Can you work these out from the model? Positions are in its coordinate system, mm. Coordinates: 2 decimals unless noted, no trailing zeros. Write each loop counter-clockwise with the first axis right and the second up, starting at its lowest first coordinate (ties: lowest second). Pieces come first, ordered by that corner, then holes. Notation, with made-up numbers: (51.25, -1) - (75.25, -1) arc R6 ccw to (75.25, 3) - close; hole circle Ø2 at (61, 72.5). An arc over 180 degrees is marked (long way). Use one line per item in the form item = value. Start each with the question number.
(1) If we section it at C-C on z = -33.5: Please give me the cut outline in (x, y).
(2) If I drill on probe 1 along X at (y, z) = (1.05, -12.5); probe 2 along X at (y, z) = (0.9, -21); probe 3 along X at (y, z) = (2.1, -23.35), over which ranges is the centre line in solid material (lowest first)? Write a range as from..to.
(3) For pin 1 Ø0.9 at (x, y) = (55, 2) entering from -Z, with a flat end and sliding along its axis, tell me the tip position at first contact or that it passes through.
(4) If we section it at B-B on z = -12.5: Please give me the cut outline in (x, y).
(5) If we section it at A-A on x = 47: Please give me the cut outline in (y, z), then the cut area to 4 significant figures.
(6) If we section it at D-D on x = 32: Please give me the cut outline in (y, z).
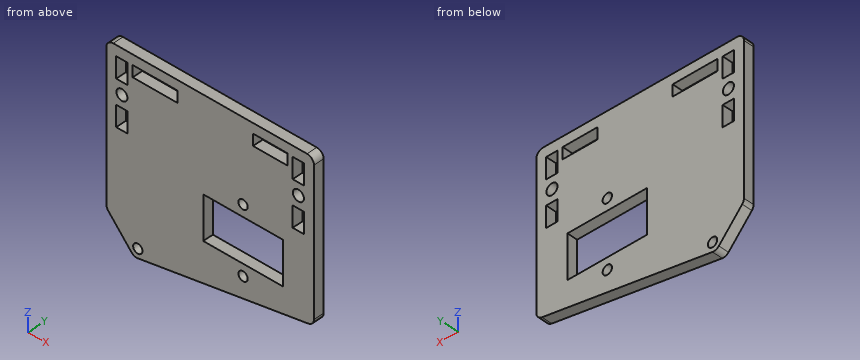
```python
from build123d import *

# Parameters (mm, degrees)
BOSS_EXTRUDE1_DEPTH = 3
SKETCH2_R           = 1.35
SKETCH2_R_2         = 1.6
SKETCH2_W           = 3
SKETCH2_H           = 6
SKETCH2_W_2         = 13
SKETCH2_H_2         = 3
SKETCH2_W_3         = 10
SKETCH2_W_4         = 23
SKETCH2_H_3         = 12.5
MAIN_HOLES_DEPTH    = 4
SKETCH3_W           = 0.15
SKETCH3_H           = 6
SKETCH3_W_2         = 10
SKETCH3_H_2         = 0.15
SKETCH3_W_3         = 13
TOLERANCE_DEPTH     = 4


with BuildPart() as part:
    # Sketch1 → Boss-Extrude1 (new body)
    with BuildSketch(Plane(origin=(0, 0, 0), x_dir=(1, 0, 0), z_dir=(0, 1, 0))):
        with BuildLine():
            Line((58.341082867, 45.287120273), (9.096557402, 53.810211219))
            ThreePointArc((9.096557402, 53.810211219), (8.095316223, 53.72741672), (7.260655898, 53.168237885))
            Line((7.260655898, 53.168237885), (0.505181363, 45.568329033))
            ThreePointArc((0.505181363, 45.568329033), (0.130556597, 44.95036247), (0, 44.239601355))
            Line((0, 44.239601355), (0, 2))
            ThreePointArc((0, 2), (0.585786438, 0.585786438), (2, 0))
            Line((2, 0), (58, 0))
            ThreePointArc((58, 0), (59.414213562, 0.585786438), (60, 2))
            Line((60, 2), (60, 43.316419261))
            ThreePointArc((60, 43.316419261), (59.530059759, 44.604408831), (58.341082867, 45.287120273))
        make_face()
    extrude(amount=BOSS_EXTRUDE1_DEPTH)

    # Sketch2 → Main Holes (cut, through all)
    with BuildSketch(Plane(origin=(0, 3, 0), x_dir=(1, 0, 0), z_dir=(0, 1, 0))):
        with Locations((9.079882179, 51.212916529)):
            Circle(SKETCH2_R)
        with Locations((39.5, 42.55)):
            Circle(SKETCH2_R)
        with Locations((39.5, 23.35)):
            Circle(SKETCH2_R)
        with Locations((55.5, 12.5)):
            Circle(SKETCH2_R_2)
        with Locations((4.5, 12.5)):
            Circle(SKETCH2_R_2)
        with Locations((4.5, 6)):
            Rectangle(SKETCH2_W, SKETCH2_H)
        with Locations((4.5, 19)):
            Rectangle(SKETCH2_W, SKETCH2_H)
        with Locations((55.5, 6)):
            Rectangle(SKETCH2_W, SKETCH2_H)
        with Locations((55.5, 19)):
            Rectangle(SKETCH2_W, SKETCH2_H)
        with Locations((14.1, 4.5)):
            Rectangle(SKETCH2_W_2, SKETCH2_H_2)
        with Locations((47.4, 4.5)):
            Rectangle(SKETCH2_W_3, SKETCH2_H_2)
        with Locations((39.5, 32.95)):
            Rectangle(SKETCH2_W_4, SKETCH2_H_3)
    extrude(amount=-MAIN_HOLES_DEPTH, mode=Mode.SUBTRACT)

    # Sketch3 → Tolerance (cut, through all)
    with BuildSketch(Plane(origin=(0, 3, 0), x_dir=(1, 0, 0), z_dir=(0, 1, 0))):
        with Locations((6.075, 19)):
            Rectangle(SKETCH3_W, SKETCH3_H)
        with Locations((2.925, 19)):
            Rectangle(SKETCH3_W, SKETCH3_H)
        with Locations((6.075, 6)):
            Rectangle(SKETCH3_W, SKETCH3_H)
        with Locations((2.925, 6)):
            Rectangle(SKETCH3_W, SKETCH3_H)
        with Locations((57.075, 6)):
            Rectangle(SKETCH3_W, SKETCH3_H)
        with Locations((53.925, 6)):
            Rectangle(SKETCH3_W, SKETCH3_H)
        with Locations((57.075, 19)):
            Rectangle(SKETCH3_W, SKETCH3_H)
        with Locations((53.925, 19)):
            Rectangle(SKETCH3_W, SKETCH3_H)
        with Locations((47.4, 6.075)):
            Rectangle(SKETCH3_W_2, SKETCH3_H_2)
        with Locations((47.4, 2.925)):
            Rectangle(SKETCH3_W_2, SKETCH3_H_2)
        with Locations((14.1, 6.075)):
            Rectangle(SKETCH3_W_3, SKETCH3_H_2)
        with Locations((14.1, 2.925)):
            Rectangle(SKETCH3_W_3, SKETCH3_H_2)
    extrude(amount=-TOLERANCE_DEPTH, mode=Mode.SUBTRACT)


solid = part.part
```
Reported:
q1.outline = (0, 0) - (28, 0) - (28, 3) - (0, 3) - close; (51, 0) - (60, 0) - (60, 3) - (51, 3) - close
q2.probe_1 = 0..2.9, 6.1..53.9, 57.1..60
q2.probe_2 = 0..2.85, 6.15..53.85, 57.15..60
q2.probe_3 = 0..38.15, 40.85..60
q3.pin_1 = -45.94
q4.outline = (0, 0) - (2.9, 0) - (2.9, 3) - (0, 3) - close; (6.1, 0) - (53.9, 0) - (53.9, 3) - (6.1, 3) - close; (57.1, 0) - (60, 0) - (60, 3) - (57.1, 3) - close
q5.outline = (0, -47.25) - (3, -47.25) - (3, -39.2) - (0, -39.2) - close; (0, -26.7) - (3, -26.7) - (3, -6.15) - (0, -6.15) - close; (0, -2.85) - (3, -2.85) - (3, 0) - (0, 0) - close
q5.area = 94.35 mm2
q6.outline = (0, -49.85) - (3, -49.85) - (3, -39.2) - (0, -39.2) - close; (0, -26.7) - (3, -26.7) - (3, 0) - (0, 0) - close
